Could you check a few things on this model? Use its own coordinates, in mm. Face numbers are marked on the shaded views. A direction names the side the tool comes from. Give positions to 0.01 mm unless a question says otherwise; leave off trailing zeros. Order: outer loops, then holes, each group sorted by start corner. A loop starts at its lowest first (then second) coordinate and runs counter-clockwise, first axis right, second up.
from build123d import *

# Parameters (mm, degrees)
SKETCH1_R           = 3.3782
BOSS_EXTRUDE1_DEPTH = 3.175


with BuildPart() as part:
    # Sketch1 → Boss-Extrude1 (new body, symmetric)
    with BuildSketch(Plane.XY):
        with BuildLine():
            Line((-19.885725358, 31.685738515), (-49.2125, 31.685738515))
            ThreePointArc((-49.2125, 31.685738515), (-53.702628061, 29.825866575), (-55.5625, 25.335738515))
            Line((-55.5625, 25.335738515), (-55.5625, -19.84375))
            ThreePointArc((-55.5625, -19.84375), (-53.702628061, -24.333878061), (-49.2125, -26.19375))
            Line((-49.2125, -26.19375), (-23.8125, -26.19375))
            ThreePointArc((-23.8125, -26.19375), (-19.322371939, -24.333878061), (-17.4625, -19.84375))
            Line((-17.4625, -19.84375), (-17.4625, 0))
            ThreePointArc((-17.4625, 0), (-1.497194511, 17.398198609), (17.205767985, 2.983362915))
            ThreePointArc((17.205767985, 2.983362915), (18.376051148, 1.93292337), (19.670597549, 2.825747839))
            ThreePointArc((19.670597549, 2.825747839), (19.745172941, 11.941624881), (14.793099056, 19.595495794))
            ThreePointArc((14.793099056, 19.595495794), (-1.415498584, 28.884168232), (-19.885725358, 31.685738515))
        make_face()
        with Locations((-35.321875, -20.32)):
            Circle(SKETCH1_R, mode=Mode.SUBTRACT)
        with Locations((-35.321875, 20.32)):
            Circle(SKETCH1_R, mode=Mode.SUBTRACT)
        with BuildLine():
            Line((-48.275875, 10.8458), (-48.275875, -10.8458))
            ThreePointArc((-48.275875, -10.8458), (-47.658397516, -12.336522516), (-46.167675, -12.954))
            Line((-46.167675, -12.954), (-24.476075, -12.954))
            ThreePointArc((-24.476075, -12.954), (-22.985352484, -12.336522516), (-22.367875, -10.8458))
            Line((-22.367875, -10.8458), (-22.367875, 10.8458))
            ThreePointArc((-22.367875, 10.8458), (-22.985352484, 12.336522516), (-24.476075, 12.954))
            Line((-24.476075, 12.954), (-46.167675, 12.954))
            ThreePointArc((-46.167675, 12.954), (-47.658397516, 12.336522516), (-48.275875, 10.8458))
        make_face(mode=Mode.SUBTRACT)
    extrude(amount=BOSS_EXTRUDE1_DEPTH, both=True)


solid = part.part
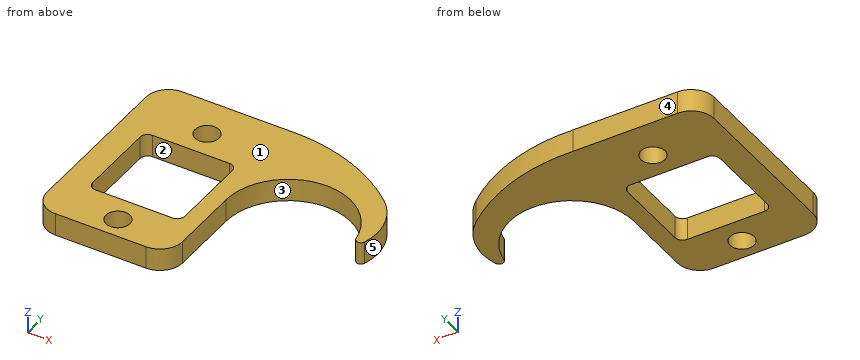
Item 1: Imagine slicing it at D-D on x = 9.5. List the corners of the cut face in (y, z) for me (3 decimals).
Findings:
outline: (14.652, -3.175) - (23.539, -3.175) - (23.539, 3.175) - (14.652, 3.175) - close
Item 2: We'd pull the mould along X, two halves only. Please class the marked faces 3, 4 and 5: +X half, -X half, draft (parallel to the pull), parting line (faces both ways), or undercut.
Findings:
face 3: undercut
face 4: draft
face 5: +X half
Item 3: For the marked faces 1 and 2, which set-ups out of +Z, -Z, +X, -X, +Y, -Y let a thin tool reach every point of the face, with its end or its side?
Findings:
face 1: +Z, +X, -X, +Y, -Y
face 2: +Z, -Z
Item 4: Imagine slicing it at A-A on z = 2.25. Give the number of separate pieces and of enclosed holes in the cut face, then the cut area to 3 significant figures.
Findings:
separate pieces: 1
enclosed holes: 3
area: 1,940 mm2
Item 5: Please list where these lines run through material, in increasing order: line 1 along Y through (x, z) = (-25, 0.5); line 2 along X through (y, z) = (4, 1.5); line 3 along Y through (x, z) = (-38, -0.5).
Findings:
line 1: y = -26.19 to -12.95, 12.95 to 31.69
line 2: x = -55.56 to -48.28, -22.37 to -17, 17 to 19.98
line 3: y = -26.19 to -22.38, -18.26 to -12.95, 12.95 to 18.26, 22.38 to 31.69
Item 6: Imagine slicing it at B-B on y = -19. List the corners of the cut face in (x, z) for me (1 decimal), then the cut area to 3 significant figures.
Findings:
outline: (-55.6, -3.2) - (-38.4, -3.2) - (-38.4, 3.2) - (-55.6, 3.2) - close; (-32.2, -3.2) - (-17.5, -3.2) - (-17.5, 3.2) - (-32.2, 3.2) - close
area: 202 mm2
Item 7: For pin 1 (3 mm diameter, centred on x = -20, z = -2.5, fed in from +Y); pin 2 (2 mm diameter, centred on y = 5, z = -1.5, fed in from +X); pin 3 (3 mm diameter, centred on y = 1, z = 0, fed in from +X), each with a flat end and sliding along its axis, tell me the tip position at first contact or that it passes through.
Findings:
pin 1: stops at y = 31.71
pin 2: stops at x = 20.31
pin 3: stops at x = 19.52
Item 8: Imagine slicing it at C-C on x = -33. List the corners of the cut face in (y, z) for me (3 decimals), then the cut area to 3 significant figures.
Findings:
outline: (-26.194, -3.175) - (-22.774, -3.175) - (-22.774, 3.175) - (-26.194, 3.175) - close; (-17.866, -3.175) - (-12.954, -3.175) - (-12.954, 3.175) - (-17.866, 3.175) - close; (12.954, -3.175) - (17.866, -3.175) - (17.866, 3.175) - (12.954, 3.175) - close; (22.774, -3.175) - (31.686, -3.175) - (31.686, 3.175) - (22.774, 3.175) - close
area: 141 mm2
